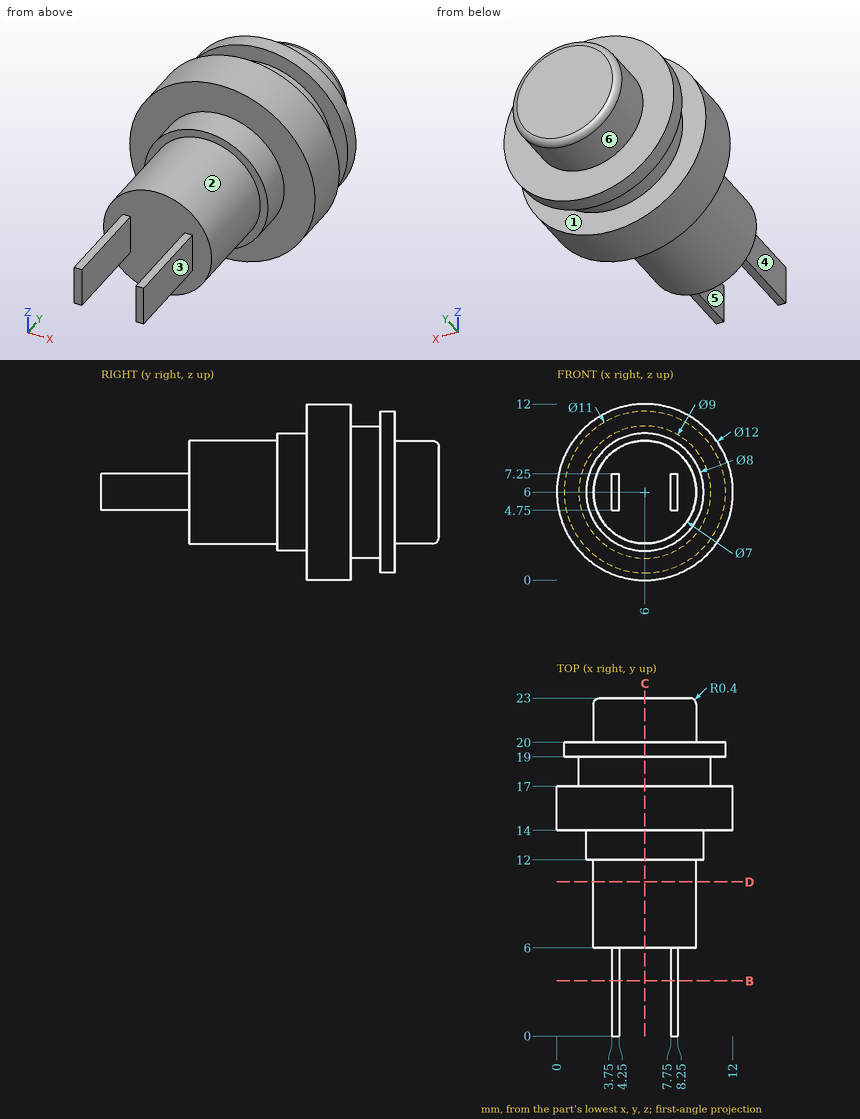
The figure shows three views and two pictorial views of one solid part (mm, origin at its lowest corner). Answer the questions. A direction names the side the tool comes from. Coordinates: 2 decimals unless noted, no trailing zeros. Write each loop counter-clockwise with the first axis right and the second up, starting at its lowest first coordinate (ties: lowest second). Pieces come first, ordered by that corner, then holes. Notation, with made-up numbers: (2, 61.25) -> (37, 61.25) arc R11 ccw to (37, 72.25) -> close; hole circle Ø3 at (5, -33.5). An arc over 180 degrees is marked (long way). Return JSON: item names as keys, results as strings.
1. A cutting plane is placed at C-C (x = 6). Determine the outline of the cut face in (y, z).
Found:
{"outline": "(6, 2.5) -> (12, 2.5) -> (12, 2) -> (14, 2) -> (14, 0) -> (17, 0) -> (17, 1.5) -> (19, 1.5) -> (19, 0.5) -> (20, 0.5) -> (20, 2.5) -> (22.6, 2.5) arc R0.4 ccw to (23, 2.9) -> (23, 9.1) arc R0.4 ccw to (22.6, 9.5) -> (20, 9.5) -> (20, 11.5) -> (19, 11.5) -> (19, 10.5) -> (17, 10.5) -> (17, 12) -> (14, 12) -> (14, 10) -> (12, 10) -> (12, 9.5) -> (6, 9.5) -> close"}
2. A cutting plane is placed at B-B (y = 3.75). Determine the outline of the cut face in (x, z), and give its area (3 significant figures).
Found:
{"outline": "(3.75, 4.75) -> (4.25, 4.75) -> (4.25, 7.25) -> (3.75, 7.25) -> close; (7.75, 4.75) -> (8.25, 4.75) -> (8.25, 7.25) -> (7.75, 7.25) -> close", "area": "2.50 mm2"}
3. A cutting plane is placed at D-D (y = 10.5). Determine the outline of the cut face in (x, z).
Found:
{"outline": "circle Ø7 at (6, 6)"}
4. A tool of negligible diameter and unlimited length cuts with its end or side. For the marked faces 1, 2 and 3, from which of +Z, -Z, +X, -X, +Y, -Y can it reach the whole face along a straight path? Write none if from no direction.
Found:
{"face 1": "none", "face 2": "-Y", "face 3": "+Z, -Z, +X, -Y"}
5. Each of these flat-tipped pins is pushed along its axis until it touches: P1, Ø6, axis at x = 2.5, z = 9, coming from the +Y side; P2, Ø5, axis at x = 9, y = 11, coming from the +Z side; P3, Ø2, axis at x = 8.5, y = 2.5, coming from the +Z side; P4, Ø0.8, axis at y = 3, z = 5.5, coming from the +X side. Where does it stop, or does it pass through?
Found:
{"P1": "y = 23", "P2": "z = 9.94", "P3": "z = 7.25", "P4": "x = 8.25"}
6. Determine the mould class of the marked faces 4, 5 and 6 for opening direction X: pulls with the +X half, pulls with the -X half, needs draft (parallel to the pull), parting line crosses it, or undercut.
Found:
{"face 4": "pulls with the -X half", "face 5": "undercut", "face 6": "parting line crosses it"}
7. Find the intervals of material crossed by line 1 along X through (y, z) = (3, 6.5); line 2 along Y through (x, z) = (4.25, 10.75); line 3 along Y through (x, z) = (5, 9.75), in increasing order. Write a range as from..to.
Found:
{"line 1": "3.75..4.25, 7.75..8.25", "line 2": "14..17, 19..20", "line 3": "12..20"}
